Geometry: final body of the model. Coordinates: model frame, mm. A direction names the side the tool comes from. Give positions to 0.01 mm unless a question says otherwise; leave off trailing zeros. Write each loop counter-clockwise with the first axis right and the second up, starting at its lowest first coordinate (ties: lowest second). Pieces come first, ordered by that corner, then holes. Notation, with made-up numbers: (16.5, -33) -> (31.5, -33) arc R12 cw to (31.5, -27) -> close; hole circle Ø3 at (38, -32). An arc over 180 degrees is marked (long way). Answer as a JSON object with one key per item and string values.
from build123d import *

# Parameters (mm, degrees)
SKETCH1_R           = 14.2875
BOSS_EXTRUDE1_DEPTH = 6.35
BOSS_EXTRUDE2_DEPTH = 6.35
CIRPATTERN1_COUNT   = 13


with BuildPart() as part:
    # Sketch1 → Boss-Extrude1 (new body)
    with BuildSketch(Plane.XY):
        Circle(SKETCH1_R)
        Polygon((7.332348419, 0), (3.666174209, 6.35), (-3.666174209, 6.35), (-7.332348419, 0), (-3.666174209, -6.35), (3.666174209, -6.35), align=None, mode=Mode.SUBTRACT)
    extrude(amount=BOSS_EXTRUDE1_DEPTH)

    # Sketch2 → Boss-Extrude2 (add)
    with BuildSketch(Plane.XY):
        Polygon((-1.27, 17.018), (1.27, 17.018), (1.905, 13.843), (-1.905, 13.843), align=None)
    boss_extrude2 = extrude(amount=BOSS_EXTRUDE2_DEPTH)

    # CirPattern1: Boss-Extrude2 ×13 about axis
    cirpattern1_axis = Axis((0, 0, 0), (0, 0, 1))
    for i in range(1, CIRPATTERN1_COUNT):
        add(boss_extrude2.rotate(cirpattern1_axis, i * 360 / CIRPATTERN1_COUNT))


solid = part.part
Q1. First-contact query: P1, Ø3, axis at y = -5.5, z = 4, coming from the -X side; P2, Ø1.9, axis at x = 0.5, z = 2, coming from the -Y side; P3, Ø4, axis at x = -11, y = -3, coming from the -Z side; P4, Ø3, axis at x = -12, z = 1, coming from the -Y side. Flat tips, straight axial feed; report the tip coordinate or a pass-through.
Values:
{"P1": "x = -16.36", "P2": "y = -14.29", "P3": "z = 0", "P4": "y = -13.43"}
Q2. Cut plane A-A (y = -4). Return the cut outline in (x, z).
Values:
{"outline": "(-15.01, 0) -> (-5.02, 0) -> (-5.02, 6.35) -> (-15.01, 6.35) -> close; (5.02, 0) -> (15.01, 0) -> (15.01, 6.35) -> (5.02, 6.35) -> close"}
Q3. Mould query, pull axis X, two halves, no side actions, for faces 1 (the flat face through (5.525, 3.131, 3.131)), 2 (the flat face through (1.55, 15.61, 3.13)), 3 (the flat face through (13.73, 7.59, 3.13)), 4 (the flat face through (-3.1, -6.5, 0)). Classes: pulls with the +X half, pulls with the -X half, needs draft (parallel to the pull), parting line crosses it, or undercut.
Values:
{"face 1": "undercut", "face 2": "undercut", "face 3": "pulls with the +X half", "face 4": "needs draft"}
Q4. Material intervals for L1, parallel to X at y = 15, z = 5; L2, parallel to X at y = 10.5, z = 1.75; L3, parallel to Y at x = 0.5, z = 2.5, sorted ascending. Write a range as from..to.
Values:
{"L1": "-8.04..-6.25, -1.67..1.67, 6.25..8.04", "L2": "-13.43..-12.79, -9.69..9.69, 12.79..13.43", "L3": "-14.28..-6.35, 6.35..17.02"}
Q5. Cut plane B-B (y = -10). Return the cut outline in (x, z).
Values:
{"outline": "(-11.13, 0) -> (11.13, 0) -> (11.13, 6.35) -> (-11.13, 6.35) -> close"}
Q6. Set-up query: faces 5 (the flat face through (5.474, -3.219, 3.131)), 6 (the flat face through (11.49, -10.62, 3.13)), 7 (the flat face through (-14.01, -6.98, 3.13)). Return all of +Z, -Z, +X, -X, +Y, -Y with unobstructed straight access to the full face (end or side cutting, diameter ignored); none if empty.
Values:
{"face 5": "+Z, -Z", "face 6": "+Z, -Z, +X", "face 7": "+Z, -Z, -Y"}
